Verification items for this drawing (mm, ordinates from the low corner). Round coordinates to 2 decimals unless told otherwise and drop trailing zeros. Loops run counter-clockwise (first coordinate to the right, second up) from the corner with the lowest first, then second, coordinate; pieces in that order, holes last. Notation, with made-up numbers: M 21,-15 L 71,-15 A19 ccw 71,-2 Z; hole C 65.25,86 d7. An arc over 180 degrees is marked long. Answer in a Markdown table with one row per item. Add a question column.
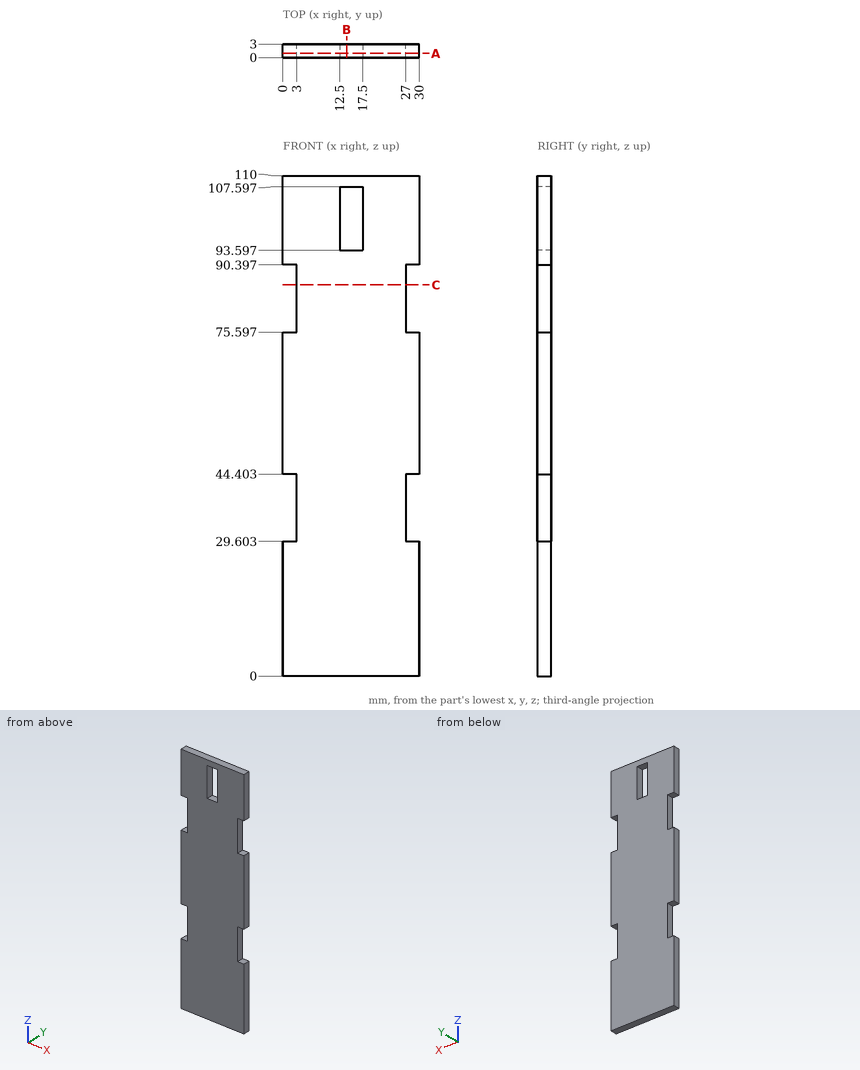
1) Cross-section at B-B, the plane x = 14. Record the boundary of the cut face in (y, z).
2) Thickness scan on L1, parallel to Z at x = 27.25, y = 1.3; L2, parallel to X at y = 0.8, z = 105; L3, parallel to X at y = 0.6, z = 36. Record the ranges inside material, lowest first. Write a range as [from, to].
3) Cross-section at A-A, the plane y = 0.95. Record the boundary of the cut face in (x, z).
4) Go/stop test with flat-tipped pins: pin 1 (0.9 mm diameter, centred on y = 1.5, z = 84.5, fed in from -X); pin 2 (1.5 mm diameter, centred on y = 1, z = 33.5, fed in from +X). Record where each tip stops, or that it passes through.
5) Cross-section at C-C, the plane z = 86. Record the boundary of the cut face in (x, y), plus the area to 3 significant figures.
Worked answers:
| question | item | result |
|---|---|---|
| 1 | outline | M 0,0 L 3,0 L 3,93.6 L 0,93.6 Z; M 0,107.6 L 3,107.6 L 3,110 L 0,110 Z |
| 2 | L1 | z = [0, 29.6], [44.4, 75.6], [90.4, 110] |
| 2 | L2 | x = [0, 12.5], [17.5, 30] |
| 2 | L3 | x = [3, 27] |
| 3 | outline | M 0,0 L 30,0 L 30,29.6 L 27,29.6 L 27,44.4 L 30,44.4 L 30,75.6 L 27,75.6 L 27,90.4 L 30,90.4 L 30,110 L 0,110 L 0,90.4 L 3,90.4 L 3,75.6 L 0,75.6 L 0,44.4 L 3,44.4 L 3,29.6 L 0,29.6 Z; hole M 12.5,93.6 L 17.5,93.6 L 17.5,107.6 L 12.5,107.6 Z |
| 4 | pin 1 | stops at x = 3 |
| 4 | pin 2 | stops at x = 27 |
| 5 | outline | M 3,0 L 27,0 L 27,3 L 3,3 Z |
| 5 | area | 72.0 mm2 |
